from build123d import *

# Parameters (mm, degrees)
F1_R     = 1.905
F2_DEPTH = 0.508
F8_DEPTH = 0.762
F9_R     = 0.762


with BuildPart() as f2:
    # F1 (on Top) → F2 (new body)
    with BuildSketch(Plane.XY):
        with BuildLine():
            ThreePointArc((19.05, 0), (17.190128, 4.490128), (12.7, 6.35))
            Line((12.7, 6.35), (-12.7, 6.35))
            ThreePointArc((-12.7, 6.35), (-17.190128, 4.490128), (-19.05, 0))
            Line((-19.05, 0), (-19.05, -6.35))
            Line((-19.05, -6.35), (19.05, -6.35))
            Line((19.05, -6.35), (19.05, 0))
        make_face()
        with Locations((-12.7, 0)):
            Circle(F1_R, mode=Mode.SUBTRACT)
        Circle(F1_R, mode=Mode.SUBTRACT)
        with Locations((12.7, 0)):
            Circle(F1_R, mode=Mode.SUBTRACT)
    extrude(amount=F2_DEPTH)

    # F7 (on offset) → F8 (join)
    with BuildSketch(Plane.XZ.offset(6.35)):
        with BuildLine():
            Line((-19.05, 6.35), (-19.05, 0))
            Line((-19.05, 0), (19.05, 0))
            Line((19.05, 0), (19.05, 6.35))
            ThreePointArc((19.05, 6.35), (17.190128, 10.840128), (12.7, 12.7))
            Line((12.7, 12.7), (-12.7, 12.7))
            ThreePointArc((-12.7, 12.7), (-17.190128, 10.840128), (-19.05, 6.35))
        make_face()
        with BuildLine():
            Line((-11.176, 8.636), (-11.176, 4.064))
            ThreePointArc((-11.176, 4.064), (-13.208, 2.032), (-15.24, 4.064))
            Line((-15.24, 4.064), (-15.24, 8.636))
            ThreePointArc((-15.24, 8.636), (-13.208, 10.668), (-11.176, 8.636))
        make_face(mode=Mode.SUBTRACT)
        with BuildLine():
            Line((-2.032, 4.064), (-2.032, 8.636))
            ThreePointArc((-2.032, 8.636), (0, 10.668), (2.032, 8.636))
            Line((2.032, 8.636), (2.032, 4.064))
            ThreePointArc((2.032, 4.064), (0, 2.032), (-2.032, 4.064))
        make_face(mode=Mode.SUBTRACT)
        with BuildLine():
            Line((15.24, 8.636), (15.24, 4.064))
            ThreePointArc((15.24, 4.064), (13.208, 2.032), (11.176, 4.064))
            Line((11.176, 4.064), (11.176, 8.636))
            ThreePointArc((11.176, 8.636), (13.208, 10.668), (15.24, 8.636))
        make_face(mode=Mode.SUBTRACT)
    extrude(amount=-F8_DEPTH)

    # F9
    f9_edges = [f2.edges().sort_by_distance(p)[0] for p in [
        (0, -6.35, 0),
    ]]
    fillet(f9_edges, radius=F9_R)


solid = f2.part
Here's how the part is built. I have some questions about the finished solid (model axes, mm). A direction names the side the tool comes from. Give positions to 0.01 mm unless a question says otherwise; leave off trailing zeros. Loops run counter-clockwise (first coordinate to the right, second up) from the corner with the lowest first, then second, coordinate; pieces in that order, holes last. Notation, with made-up numbers: (44, 70) -> (72, 70) arc R30 cw to (72, 97) -> close; hole circle Ø6 at (54.5, 83). An arc over 180 degrees is marked (long way). Answer as a JSON object with one key per item and string values. Group by question number.
Item 1: On a 3-axis mill with a long thin cutter (end or side, diameter ignored), from which of +Z, -Z, +X, -X, +Y, -Y can I reach the whole of each face in a straight line? I mean faces 1 (the flat face through (19.05, -6, 2)), 2 (the flat face through (0, -5.588, 11)), 3 (the cylindrical face through (-13.253, -5.974, 10.668)). Say none if no direction works.
Item 2: Imagine slicing it at A-A on z = 5.5. Write out the boundary of the cut face in (x, y), then the cut area to 3 significant figures.
Item 3: Thinking about a two-plate mould opening in Z: for faces 4 (the cylindrical face through (-17.14, -5.97, 10.89)), 5 (the cylindrical face through (0.045, -5.974, 2.032)), 6 (the cylindrical face through (-13.163, -5.974, 2.032)), 7 (the flat face through (-0.3, -2.2, 0)), which applies, pulls with the +Z half, pulls with the -Z half, needs draft (parallel to the pull), parting line crosses it, or undercut?
Item 4: Will these pins go through, and if not, where does the flat tip stop? pin 1 (4 mm diameter, centred on y = -3, z = 10.5, fed in from +X); pin 2 (1 mm diameter, centred on x = 11, y = 0.5, fed in from +Z); pin 3 (1.5 mm diameter, centred on x = -7.5, z = 9.5, fed in from +Y).
Item 5: Imagine slicing it at B-B on x = 0. Write out the boundary of the cut face in (y, z) (3 decimals), then the cut area to 3 significant figures.
Item 6: I need wall thicknesses on L1, parallel to Y at x = -5, z = 4; L2, parallel to Z at x = 4, y = 3.5; L3, parallel to Y at x = 0, z = 0.3 (3 decimals). Which ranges of each line are inside material? Lowest first, please.
Item 7: Imagine slicing it at C-C on z = 7.75. Write out the boundary of the cut face in (x, y).
Item 8: Imagine slicing it at D-D on y = 3. Write out the boundary of the cut face in (x, z), then the cut area to 3 significant figures.
Answer list:
{
 "1": {"face 1": "+Z, -Z, +X, +Y, -Y", "face 2": "+Z, +X, -X, +Y", "face 3": "+Y, -Y"},
 "2": {"outline": "(-19.05, -6.35) -> (-15.24, -6.35) -> (-15.24, -5.59) -> (-19.05, -5.59) -> close; (-11.18, -6.35) -> (-2.03, -6.35) -> (-2.03, -5.59) -> (-11.18, -5.59) -> close; (2.03, -6.35) -> (11.18, -6.35) -> (11.18, -5.59) -> (2.03, -5.59) -> close; (15.24, -6.35) -> (19.05, -6.35) -> (19.05, -5.59) -> (15.24, -5.59) -> close", "area": "19.7 mm2"},
 "3": {"face 4": "pulls with the +Z half", "face 5": "undercut", "face 6": "undercut", "face 7": "pulls with the -Z half"},
 "4": {"pin 1": "passes through", "pin 2": "stops at z = 0.51", "pin 3": "stops at y = -5.59"},
 "5": {"outline": "(-6.35, 0.762) arc R0.762 ccw to (-5.588, 0) -> (-1.905, 0) -> (-1.905, 0.508) -> (-5.588, 0.508) -> (-5.588, 2.032) -> (-6.35, 2.032) -> close; (-6.35, 10.668) -> (-5.588, 10.668) -> (-5.588, 12.7) -> (-6.35, 12.7) -> close; (1.905, 0) -> (6.35, 0) -> (6.35, 0.508) -> (1.905, 0.508) -> close", "area": "7.10 mm2"},
 "6": {"L1": "y = -6.35 to -5.59", "L2": "z = 0 to 0.51", "L3": "y = -6.194 to -1.905, 1.905 to 6.35"},
 "7": {"outline": "(-18.89, -6.35) -> (-15.24, -6.35) -> (-15.24, -5.59) -> (-18.89, -5.59) -> close; (-11.18, -6.35) -> (-2.03, -6.35) -> (-2.03, -5.59) -> (-11.18, -5.59) -> close; (2.03, -6.35) -> (11.18, -6.35) -> (11.18, -5.59) -> (2.03, -5.59) -> close; (15.24, -6.35) -> (18.89, -6.35) -> (18.89, -5.59) -> (15.24, -5.59) -> close"},
 "8": {"outline": "(-18.3, 0) -> (18.3, 0) -> (18.3, 0.51) -> (-18.3, 0.51) -> close", "area": "18.6 mm2"}
}
